Verification items for the finished model (mm, model axes). Face numbers are marked on the shaded views. A direction names the side the tool comes from. Round coordinates to 2 decimals unless told otherwise and drop trailing zeros. Order: outer loops, then holes, each group sorted by start corner. A loop starts at its lowest first (then second) coordinate and runs counter-clockwise, first axis right, second up. Notation, with made-up numbers: (12, 23) -> (61, 23) arc R5 cw to (61, 28) -> close; hole circle Ø11 at (19.25, 0.5). An arc over 180 degrees is marked (long way). Put each result on its own line as item: value.
from build123d import *

# Parameters (mm, degrees)
BOSS_EXTRUDE1_DEPTH             = 10
BOSS_EXTRUDE2_DEPTH             = 9
CBORE_FOR_M5_SBHCS1_D           = 5.5
CBORE_FOR_M5_SBHCS1_CBORE_D     = 10.5
CBORE_FOR_M5_SBHCS1_CBORE_DEPTH = 2.75
CBORE_FOR_M5_SBHCS2_D           = 5.5
CBORE_FOR_M5_SBHCS2_CBORE_D     = 10.5
CBORE_FOR_M5_SBHCS2_CBORE_DEPTH = 2.75
CBORE_FOR_M3_SBHCS1_D           = 3.4
CBORE_FOR_M3_SBHCS1_CBORE_D     = 6.7
CBORE_FOR_M3_SBHCS1_CBORE_DEPTH = 16
CBORE_FOR_M3_SBHCS2_D           = 3.4
CBORE_FOR_M3_SBHCS2_CBORE_D     = 6.7
CBORE_FOR_M3_SBHCS2_CBORE_DEPTH = 6
F_5_4_5_4_DIAMETER_HOLE1_D      = 5.4
FILLET3_R                       = 9


with BuildPart() as part:
    # Sketch1 → Boss-Extrude1 (new body)
    with BuildSketch(Plane(origin=(0, 0, 0), x_dir=(1, 0, 0), z_dir=(0, 1, 0))):
        Polygon((0, 0), (60, 0), (60, 40), (20, 40), (20, 20), (0, 20), align=None)
    extrude(amount=BOSS_EXTRUDE1_DEPTH)

    # Sketch2 → Boss-Extrude2 (add)
    with BuildSketch(Plane(origin=(0, 10, 0), x_dir=(1, 0, 0), z_dir=(0, 1, 0))):
        Polygon((20, 40), (7, 40), (7, 20), (0, 20), (0, 0), (60, 0), (60, 40), align=None)
    extrude(amount=BOSS_EXTRUDE2_DEPTH)

    # CBORE for M5 SBHCS1 (through all)
    with Locations(Plane(origin=(0, 19, 0), x_dir=(1, 0, 0), z_dir=(0, 1, 0))):
        with Locations((10, 7.5), (30, 7.5), (30, 32.5)):
            CounterBoreHole(CBORE_FOR_M5_SBHCS1_D / 2, CBORE_FOR_M5_SBHCS1_CBORE_D / 2, CBORE_FOR_M5_SBHCS1_CBORE_DEPTH)

    # CBORE for M5 SBHCS2 (through all)
    with Locations(Plane(origin=(0, 19, 0), x_dir=(1, 0, 0), z_dir=(0, 1, 0))):
        with Locations((52.5, 30), (52.5, 10)):
            CounterBoreHole(CBORE_FOR_M5_SBHCS2_D / 2, CBORE_FOR_M5_SBHCS2_CBORE_D / 2, CBORE_FOR_M5_SBHCS2_CBORE_DEPTH)

    # CBORE for M3 SBHCS1 (through all)
    with Locations(Plane(origin=(0, 0, 0), x_dir=(-1, 0, 0), z_dir=(0, -1, 0))):
        with Locations((-30, 20)):
            CounterBoreHole(CBORE_FOR_M3_SBHCS1_D / 2, CBORE_FOR_M3_SBHCS1_CBORE_D / 2, CBORE_FOR_M3_SBHCS1_CBORE_DEPTH)

    # CBORE for M3 SBHCS2 (through all)
    with Locations(Plane(origin=(0, 10, 0), x_dir=(-1, 0, 0), z_dir=(0, -1, 0))):
        with Locations((-13.5, 33)):
            CounterBoreHole(CBORE_FOR_M3_SBHCS2_D / 2, CBORE_FOR_M3_SBHCS2_CBORE_D / 2, CBORE_FOR_M3_SBHCS2_CBORE_DEPTH)

    # Ø5.4 (5.4) Diameter Hole1 (through all)
    with Locations(Plane(origin=(0, 0, 0), x_dir=(-1, 0, 0), z_dir=(0, -1, 0))):
        with Locations((-13.5, 20)):
            Hole(F_5_4_5_4_DIAMETER_HOLE1_D / 2)

    # Fillet3
    # the kernel refuses this fillet: 9 mm, written as the material it adds along each edge
    with BuildSketch(Plane(origin=(20, 10, -40), x_dir=(0, -1, 0), z_dir=(0, 0, 1))) as fillet3_piece_1_section:
        with BuildLine():
            CenterArc((FILLET3_R, -FILLET3_R), FILLET3_R, 90, 90)
            Line((0, -FILLET3_R), (0, 0))
            Line((0, 0), (FILLET3_R, 0))
        make_face()
    fillet3_piece_1 = extrude(amount=20, mode=Mode.PRIVATE)
    fillet3_piece_1 = fillet3_piece_1 - Plane(origin=(13.5, 7.877517224, -20), x_dir=(1, 0, 0), z_dir=(0, 1, 0)) * Cylinder(2.7, 76, mode=Mode.PRIVATE)
    fillet3_piece_1 = fillet3_piece_1 - Plane(origin=(13.5, 7.877517224, -33), x_dir=(-1, 0, 0), z_dir=(0, -1, 0)) * Cylinder(3.35, 76, mode=Mode.PRIVATE)
    add(fillet3_piece_1)
    with BuildSketch(Plane(origin=(33.3, 10, -20), x_dir=(0, -1, 0), z_dir=(-1, 0, 0))) as fillet3_piece_2_section:
        with BuildLine():
            CenterArc((FILLET3_R, -FILLET3_R), FILLET3_R, 90, 90)
            Line((0, -FILLET3_R), (0, 0))
            Line((0, 0), (FILLET3_R, 0))
        make_face()
    fillet3_piece_2 = extrude(amount=26.3, mode=Mode.PRIVATE)
    fillet3_piece_2 = fillet3_piece_2 - Plane(origin=(13.5, 3.343699997, -20), x_dir=(1, 0, 0), z_dir=(0, 1, 0)) * Cylinder(2.7, 89, mode=Mode.PRIVATE)
    fillet3_piece_2 = split(fillet3_piece_2, bisect_by=Plane(origin=(20, 3.343699997, -20.253192533), z_dir=(-1, 0, 0)), keep=Keep.TOP, mode=Mode.PRIVATE)
    add(fillet3_piece_2)


solid = part.part
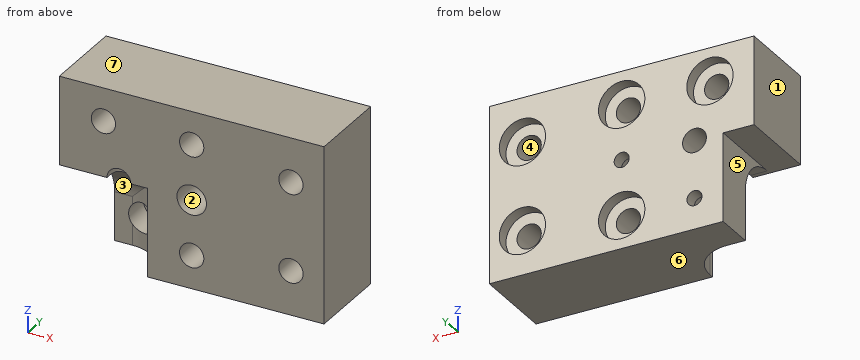
Item 1: Release check for a two-part mould opening along Z. For the marked faces 4, 5, 6 and 7 record: +Z half, -Z half, draft (parallel to the pull), parting line (faces both ways), or undercut.
Check sheet entries:
face 4: undercut
face 5: draft
face 6: -Z half
face 7: +Z half
Item 2: Section check D-D on y = 7. Record the boundary of the cut face in (x, z).
Check sheet entries:
outline: (0, -20) -> (7, -20) -> (7, -22.29) -> (12.07, -22.29) arc R2.7 cw (long way) to (14.93, -22.29) -> (17.71, -22.29) -> (17.71, -40) -> (60, -40) -> (60, 0) -> (0, 0) -> close; hole circle Ø5.5 at (10, -7.5); hole circle Ø6.7 at (30, -20); hole circle Ø5.5 at (30, -32.5); hole circle Ø5.5 at (30, -7.5); hole circle Ø5.5 at (52.5, -30); hole circle Ø5.5 at (52.5, -10)
Item 3: Section check C-C on y = 12.5. State how many separate pieces and enclosed holes the cut face has, then the cut area to 3 significant figures.
Check sheet entries:
separate pieces: 1
enclosed holes: 8
area: 2,050 mm^2
Item 4: Section check B-B on z = -11. Record the boundary of the cut face in (x, y).
Check sheet entries:
outline: (0, 0) -> (49.94, 0) -> (49.94, 16.25) -> (47.35, 16.25) -> (47.35, 19) -> (33.91, 19) -> (33.91, 16.25) -> (26.09, 16.25) -> (26.09, 19) -> (13.91, 19) -> (13.91, 16.25) -> (6.09, 16.25) -> (6.09, 19) -> (0, 19) -> close; (55.06, 0) -> (60, 0) -> (60, 19) -> (57.65, 19) -> (57.65, 16.25) -> (55.06, 16.25) -> close
Item 5: Tool access check on the marked faces 1, 2 and 3. Record the directions out of +Z, -Z, +X, -X, +Y, -Y that give a thin tool (end or side, any length) a straight path to the whole face; none if there is none.
Check sheet entries:
face 1: +Z, -Z, -X, +Y, -Y
face 2: -Y
face 3: -Z, -X, -Y
Item 6: Section check A-A on x = 52.5. Record the boundary of the cut face in (y, z), then the cut area to 4 significant figures.
Check sheet entries:
outline: (0, -40) -> (19, -40) -> (19, -35.25) -> (16.25, -35.25) -> (16.25, -32.75) -> (0, -32.75) -> close; (0, -27.25) -> (16.25, -27.25) -> (16.25, -24.75) -> (19, -24.75) -> (19, -15.25) -> (16.25, -15.25) -> (16.25, -12.75) -> (0, -12.75) -> close; (0, -7.25) -> (16.25, -7.25) -> (16.25, -4.75) -> (19, -4.75) -> (19, 0) -> (0, 0) -> close
area: 523.5 mm^2
Item 7: Material ranges on L1, parallel to Z at x = 52.5, y = 18.2; L2, parallel to Z at x = 30, y = 9.5; L3, parallel to Z at x = 30, y = 17.9, recorded low to high. Write a range as [from, to].
Check sheet entries:
L1: z = [-40, -35.25], [-24.75, -15.25], [-4.75, 0]
L2: z = [-40, -35.25], [-29.75, -23.35], [-16.65, -10.25], [-4.75, 0]
L3: z = [-40, -37.75], [-27.25, -21.7], [-18.3, -12.75], [-2.25, 0]
Item 8: Gauge pin test, flat ends, axial feed: pin 1 Ø11.5 at (x, z) = (29, -6.5) entering from +Y; pin 2 Ø5 at (y, z) = (16.5, -29) entering from -X; pin 3 Ø8.5 at (x, z) = (52.5, -30) entering from +Y; pin 4 Ø1.2 at (x, z) = (9.5, -34) entering from -Y. Record the tip position at first contact, or that the pin passes through.
Check sheet entries:
pin 1: stops at y = 19
pin 2: stops at x = 7
pin 3: stops at y = 16.25
pin 4: stops at y = 10
